Geometry check sheet. Reference: the model listing, model coordinates, mm. A direction names the side the tool comes from. Coordinates: 2 decimals unless noted, no trailing zeros. Loops run counter-clockwise (first coordinate to the right, second up) from the corner with the lowest first, then second, coordinate; pieces in that order, holes last. Notation, with made-up numbers: (83.5, 48.5) - (112.5, 48.5) arc R21 ccw to (112.5, 87.5) - close; hole circle Ø4 at (27.5, 41). An arc over 180 degrees is marked (long way). Write each question's results on one line, items separated by ' | '. Start each with the question number.
(1) Sectioned sample at B-B (x = 0). Enter the section's corners in (y, z), plus the area to 3 significant figures.
(2) Access from +Z, -Z, +X, -X, +Y, -Y to the whole of each face (thin tool, end or side, straight path). Record for faces 1 (the face through (-4.693, -1, -14)), 2 (the face through (5.307, -1, -14)), 3 (the face through (5.307, -1, 14)).
(3) Material ranges on probe 1 along X at (y, z) = (-1.9, -15); probe 2 along X at (y, z) = (13, 0); probe 3 along Z at (x, y) = (6.5, 30), recorded low to high.
(4) Sectioned sample at C-C (x = -5.75). Enter the section's corners in (y, z), plus the area to 3 significant figures.
(5) Sectioned sample at A-A (z = -15). Enter the section's corners in (x, y), plus the area to 3 significant figures.
(6) Sectioned sample at D-D (y = 11). Enter the section's corners in (x, z).
(7) Go/stop test with flat-tipped pins: pin 1 Ø5 at (x, z) = (1.5, 16) entering from +Y; pin 2 Ø3 at (x, y) = (7.5, 14.5) entering from +Z; pin 3 Ø5 at (x, y) = (4.5, 30.5) entering from -Z. Record where each tip stops, or that it passes through.
from build123d import *

# Parameters (mm, degrees)
ESQUISSE1_R        = 7.5
ESQUISSE1_R_2      = 1.65
BOSS_EXTRU_1_DEPTH = 3
BOSS_EXTRU_2_START = 58
ESQUISSE2_R        = 10
ESQUISSE2_R_2      = 7.5
BOSS_EXTRU_2_DEPTH = 58


with BuildPart() as part:
    # Esquisse1 → Boss.-Extru.1 (new body)
    with BuildSketch(Plane(origin=(0, 0, 0), x_dir=(1, 0, 0), z_dir=(0, 1, 0))):
        with BuildLine():
            Line((0, 20), (5.307172847, 20))
            Line((5.307172847, 20), (5.307172847, 8.475489152))
            ThreePointArc((5.307172847, 8.475489152), (10, 0), (5.307172847, -8.475489152))
            Line((5.307172847, -8.475489152), (5.307172847, -20))
            Line((5.307172847, -20), (0, -20))
            Line((0, -20), (-4.692827153, -20))
            Line((-4.692827153, -20), (-4.692827153, -8.830479789))
            ThreePointArc((-4.692827153, -8.830479789), (-10, 0), (-4.692827153, 8.830479789))
            Line((-4.692827153, 8.830479789), (-4.692827153, 20))
            Line((-4.692827153, 20), (0, 20))
        make_face()
        with Locations(Location((0, 0, 0), (0, 0, 270))):
            Circle(ESQUISSE1_R, mode=Mode.SUBTRACT)
        with Locations(Location((0, 15, 0), (0, 0, 270))):
            Circle(ESQUISSE1_R_2, mode=Mode.SUBTRACT)
        with Locations(Location((0, -15, 0), (0, 0, 270))):
            Circle(ESQUISSE1_R_2, mode=Mode.SUBTRACT)
    extrude(amount=-BOSS_EXTRU_1_DEPTH)

    # Esquisse2 → Boss.-Extru.2 (add)
    with BuildSketch(Plane(origin=(0, 0, 0), x_dir=(1, 0, 0), z_dir=(0, 1, 0)).offset(BOSS_EXTRU_2_START)):
        with Locations(Location((0, 0, 0), (0, 0, 270))):
            Circle(ESQUISSE2_R)
        with Locations(Location((0, 0, 0), (0, 0, 270))):
            Circle(ESQUISSE2_R_2, mode=Mode.SUBTRACT)
    extrude(amount=-BOSS_EXTRU_2_DEPTH)


solid = part.part
Outcome:
1) outline: (-3, -20) - (0, -20) - (0, -16.65) - (-3, -16.65) - close; (-3, -13.35) - (0, -13.35) - (0, -10) - (58, -10) - (58, -7.5) - (-3, -7.5) - close; (-3, 7.5) - (58, 7.5) - (58, 10) - (0, 10) - (0, 13.35) - (-3, 13.35) - close; (-3, 16.65) - (0, 16.65) - (0, 20) - (-3, 20) - close | area: 345 mm2
2) face 1: -Z, -X, +Y, -Y | face 2: -Z, +X, +Y, -Y | face 3: +Z, +X, +Y, -Y
3) probe 1: x = -4.69 to -1.65, 1.65 to 5.31 | probe 2: x = -10 to -7.5, 7.5 to 10 | probe 3: z = -7.6 to -3.74, 3.74 to 7.6
4) outline: (-3, -8.18) - (58, -8.18) - (58, -4.82) - (-3, -4.82) - close; (-3, 4.82) - (58, 4.82) - (58, 8.18) - (-3, 8.18) - close | area: 411 mm2
5) outline: (-4.69, -3) - (-1.65, -3) - (-1.65, 0) - (-4.69, 0) - close; (1.65, -3) - (5.31, -3) - (5.31, 0) - (1.65, 0) - close | area: 20.1 mm2
6) outline: circle Ø20 at (0, 0); hole circle Ø15 at (0, 0)
7) pin 1: stops at y = 0 | pin 2: stops at z = 8 | pin 3: stops at z = -9.8
